Here's how the part is built. I have some questions about the finished solid (model axes, mm). A direction names the side the tool comes from. Coordinates: 2 decimals unless noted, no trailing zeros. Write each loop counter-clockwise with the first axis right and the second up, starting at its lowest first coordinate (ties: lowest second). Pieces come first, ordered by that corner, then holes.
from build123d import *

# Parameters (mm, degrees)
CYLINDER002_R     = 2.8
CYLINDER002_DEPTH = 2.5
CYLINDER001_R     = 2.8
CYLINDER001_DEPTH = 2.5
CYLINDER003_R     = 2.8
CYLINDER003_DEPTH = 2.5
CYLINDER_R        = 2.8
CYLINDER_DEPTH    = 2.5
BOX_W             = 150
BOX_H             = 23
BOX_DEPTH         = 3


with BuildPart() as cylinder002:
    # Cylinder002 → Cylinder002 (new body)
    with BuildSketch(Plane(origin=(126, 11.5, 0.5), x_dir=(1, 0, 0), z_dir=(0, 0, 1))):
        Circle(CYLINDER002_R)
    extrude(amount=CYLINDER002_DEPTH)


with BuildPart() as cylinder001:
    # Cylinder001 → Cylinder001 (new body)
    with BuildSketch(Plane(origin=(24, 11.5, 0.5), x_dir=(1, 0, 0), z_dir=(0, 0, 1))):
        Circle(CYLINDER001_R)
    extrude(amount=CYLINDER001_DEPTH)


with BuildPart() as cylinder003:
    # Cylinder003 → Cylinder003 (new body)
    with BuildSketch(Plane(origin=(134, 11.5, 0.5), x_dir=(1, 0, 0), z_dir=(0, 0, 1))):
        Circle(CYLINDER003_R)
    extrude(amount=CYLINDER003_DEPTH)


with BuildPart() as fusion:
    # Cylinder → Cylinder (new body)
    with BuildSketch(Plane(origin=(16, 11.5, 0.5), x_dir=(1, 0, 0), z_dir=(0, 0, 1))):
        Circle(CYLINDER_R)
    extrude(amount=CYLINDER_DEPTH)

    # Fusion: union Cylinder002, Cylinder001, Cylinder003
    add(cylinder002.part)
    add(cylinder001.part)
    add(cylinder003.part)


with BuildPart() as cone:
    # Cone → Cone (revolve)
    with BuildSketch(Plane(origin=(40, 11.5, 3), x_dir=(1, 0, 0), z_dir=(0, -1, 0))):
        Polygon((0, 0), (5, 0), (1, 4), (0, 4), align=None)
    revolve(axis=Axis((40, 11.5, 3), (0, 0, 1)))


with BuildPart() as base:
    # Box → Box (new body)
    with BuildSketch(Plane.XY):
        with Locations((75, 11.5)):
            Rectangle(BOX_W, BOX_H)
    extrude(amount=BOX_DEPTH)


with BuildPart() as bottom:
    # Cone001 → Cone001 (revolve)
    with BuildSketch(Plane(origin=(110, 11.5, 3), x_dir=(1, 0, 0), z_dir=(0, -1, 0))):
        Polygon((0, 0), (5, 0), (1, 4), (0, 4), align=None)
    revolve(axis=Axis((110, 11.5, 3), (0, 0, 1)))

    # Fusion001: union Cone, base
    add(cone.part)
    add(base.part)

    # Cut: cut Fusion
    add(fusion.part, mode=Mode.SUBTRACT)


solid = bottom.part
1. On a 3-axis mill with a long thin cutter (end or side, diameter ignored), from which of +Z, -Z, +X, -X, +Y, -Y can I reach the whole of each face in a straight line? I mean faces 4 (the face through (128.67, 12.34, 1.73)), 5 (the face through (74, 12, 0)). Say none if no direction works.
2. If I drill on line 1 (Y direction, x = 126, z = 2.1); line 2 (Z direction, x = 45.5, y = 9.25); line 3 (X direction, y = 12.5, z = 5), over which ranges is the centre line in solid material (lowest first)?
3. I want a section at B-B (y = 18). List the corners of the cut face in (x, z) for me, then the cut area to 3 significant figures.
4. I want a section at D-D (x = 71.5). List the corners of the cut face in (y, z) for me, then the cut area to 3 significant figures.
5. I want a section at A-A (x = 24). List the corners of the cut face in (y, z) for me, then the cut area to 3 significant figures.
6. I want a section at C-C (x = 133). List the corners of the cut face in (y, z) for me, then the cut area to 3 significant figures.
7. Thinking about a two-plate mould opening in Y: for faces 1 (the face through (16, 12, 0.5)), 2 (the face through (150, 11, 1)), 3 (the face through (74, 23, 1)), which applies, pulls with the +Y half, pulls with the -Y half, needs draft (parallel to the pull), parting line crosses it, or undercut?
8. For pin 1 Ø1.5 at (y, z) = (5.5, 3.5) entering from +X; pin 2 Ø3 at (x, y) = (126, 12.5) entering from +Z; pin 3 Ø3 at (x, y) = (25, 12.5) entering from +Z; pin 4 Ø3 at (y, z) = (8, 5.5) entering from +X, each with a flat end and sliding along its axis, tell me the tip position at first contact or that it passes through.
Response values:
1. face 4: +Z
1. face 5: -Z, +X, -X, +Y, -Y
2. line 1: y = 0 to 8.7, 14.3 to 23
2. line 2: z = 0 to 3
2. line 3: x = 37.17 to 42.83, 107.17 to 112.83
3. outline: (0, 0) - (150, 0) - (150, 3) - (0, 3) - close
3. area: 450 mm2
4. outline: (0, 0) - (23, 0) - (23, 3) - (0, 3) - close
4. area: 69.0 mm2
5. outline: (0, 0) - (23, 0) - (23, 3) - (14.3, 3) - (14.3, 0.5) - (8.7, 0.5) - (8.7, 3) - (0, 3) - close
5. area: 55.0 mm2
6. outline: (0, 0) - (23, 0) - (23, 3) - (14.12, 3) - (14.12, 0.5) - (8.88, 0.5) - (8.88, 3) - (0, 3) - close
6. area: 55.9 mm2
7. face 1: undercut
7. face 2: needs draft
7. face 3: pulls with the +Y half
8. pin 1: stops at x = 150
8. pin 2: stops at z = 0.5
8. pin 3: stops at z = 3
8. pin 4: stops at x = 112.63
